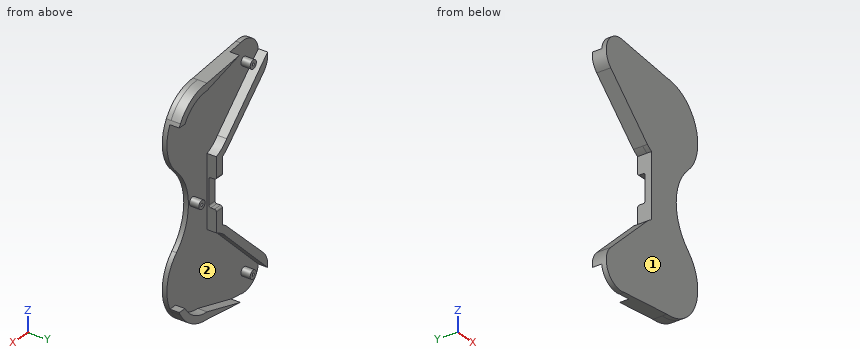
Autodesk Inventor part; units mm, degrees
ref_plane "YZ Plane" through (0, 0, 0) normal (1, 0, 0) x (0, 1, 0)
ref_plane "XZ Plane" through (0, 0, 0) normal (0, 1, 0) x (-1, 0, 0)
ref_plane "XY Plane" through (0, 0, 0) normal (0, 0, 1) x (1, 0, 0)
sketch "Boceto1" plane through (0, 0, 0) normal (0, 1, 0) x (-1, 0, 0)
  line L0 (16, -33) -> (103.2837, -54.9444)
  line L1 (38.5, 50.9711) -> (38.5, 119.0289)
  line L2 (-22.9711, -10.5) -> (-52.9711, -10.5)
  arc A0 (-22.9711, -10.5) -> (16, -33) centre (16, 12) ccw
  arc A1 (-51.515, 38.5517) -> (-6.5, 85) centre (-52.9711, 85) ccw
  arc A2 (-22.9711, -10.5) -> (16, -33) centre (16, 12) ccw
  arc A3 (-51.515, 38.5517) -> (-52.9711, -10.5) centre (16, 12) ccw
  line L3 (38.5, 50.9711) -> (38.5, 85)
  arc A4 (103.2837, -54.9444) -> (115.3375, -21.0974) centre (95.2119, -33) ccw
  line L4 (115.3375, -21.0974) -> (44.6515, 46.7)
  line L5 (16, 203) -> (103.2837, 224.9444)
  arc A5 (16, 203) -> (-22.9711, 180.5) centre (16, 158) ccw
  line L6 (115.3375, 191.0974) -> (44.6515, 123.3)
  arc A6 (115.3375, 191.0974) -> (103.2837, 224.9444) centre (95.2119, 203) ccw
  arc A7 (16, 203) -> (-22.9711, 180.5) centre (16, 158) ccw
  line L7 (38.5, 119.0289) -> (38.5, 50.9711)
  line L8 (-22.9711, 180.5) -> (-52.9711, 180.5)
  line L9 (38.5, 119.0289) -> (38.5, 85)
  arc A8 (-52.9711, 180.5) -> (-51.515, 131.4483) centre (16, 158) ccw
  arc A9 (-6.5, 85) -> (-51.515, 131.4483) centre (-52.9711, 85) ccw
  arc A10 (-22.9711, -10.5) -> (16, -33) centre (16, 12) ccw
  arc A11 (49.4751, 42.0735) -> (38.5, 50.9711) centre (16, 12) ccw
  arc A12 (38.5, 119.0289) -> (49.4751, 127.9265) centre (16, 158) ccw
  arc A13 (16, 203) -> (-22.9711, 180.5) centre (16, 158) ccw
  circle A14 centre (83.6139, -19.9457) radius 1.5
  circle A15 centre (8.5, 85) radius 1.5
  circle A16 centre (83.6139, 189.9457) radius 1.5
  arc A17 (88.6874, -45.3867) -> (105.0119, -23.002) centre (95.2119, -33) ccw
  arc A18 (105.0119, 193.002) -> (91.4604, 216.488) centre (95.2119, 203) ccw
  arc A19 (-48.2434, 32.7133) -> (-48.2434, 137.2867) centre (-52.9711, 85) ccw
  arc A20 (-48.7329, 177.1284) -> (-48.2434, 137.2867) centre (16, 158) ccw
  arc A21 (-48.2434, 32.7133) -> (-48.7329, -7.1284) centre (16, 12) ccw
  line L10 (-48.7329, -7.1284) -> (-16.2545, -7.1284)
  line L11 (-48.7329, 177.1284) -> (-16.2545, 177.1284)
  line L12 (16, 195.5) -> (91.4604, 216.488)
  line L13 (16, -25.5) -> (88.6874, -45.3867)
  line L14 (39.4427, 41.2693) -> (105.0119, -23.002)
  line L15 (105.0119, 193.002) -> (44.7948, 133.9769)
  line L16 (29.5774, 46.9558) -> (29.5774, 123.0442)
  arc A22 (44.7948, 36.0231) -> (29.5774, 46.9558) centre (16, 12) ccw
  arc A23 (-16.2545, -7.1284) -> (16, -25.5) centre (16, 12) ccw
  arc A24 (29.5774, 123.0442) -> (44.7948, 133.9769) centre (16, 158) ccw
  arc A25 (16, 195.5) -> (-16.2545, 177.1284) centre (16, 158) ccw
  circle A26 centre (83.6139, -19.9457) radius 4.5
  circle A27 centre (8.5, 85) radius 4.5
  circle A28 centre (83.6139, 189.9457) radius 4.5
  point P0 (0, 0)
  dimension "d8" = 9
  dimension "d9" = 9
  dimension "d10" = 9
extrude "Extrusión1" add sketch "Boceto1" along normal blind 10 contours A0 L2 A3 A1 A9 A8 L8 A5 L5 A6 L6 A12 L1 A11 L4 A4 L0 | A26 | A27 | A28
sketch "Boceto2" plane through (0, 0, 0) normal (0, -1, 0) x (1, 0, 0)
  line L0 (-16, 203) -> (-103.2837, 224.9444)
  line L1 (22.9711, 180.5) -> (52.9711, 180.5)
  arc A0 (22.9711, 180.5) -> (-16, 203) centre (-16, 158) ccw
  arc A1 (22.9711, 180.5) -> (-16, 203) centre (-16, 158) ccw
  arc A2 (51.515, 131.4483) -> (52.9711, 180.5) centre (-16, 158) ccw
  line L2 (-38.5, 119.0289) -> (-38.5, 85)
  arc A3 (-103.2837, 224.9444) -> (-115.3375, 191.0974) centre (-95.2119, 203) ccw
  line L3 (-115.3375, 191.0974) -> (-44.6515, 123.3)
  line L4 (-16, -33) -> (-103.2837, -54.9444)
  arc A4 (-16, -33) -> (22.9711, -10.5) centre (-16, 12) ccw
  line L5 (-115.3375, -21.0974) -> (-44.6515, 46.7)
  arc A5 (-115.3375, -21.0974) -> (-103.2837, -54.9444) centre (-95.2119, -33) ccw
  arc A6 (-16, -33) -> (22.9711, -10.5) centre (-16, 12) ccw
  line L6 (22.9711, -10.5) -> (52.9711, -10.5)
  line L7 (-38.5, 50.9711) -> (-38.5, 85)
  arc A7 (52.9711, -10.5) -> (51.515, 38.5517) centre (-16, 12) ccw
  arc A8 (51.515, 131.4483) -> (52.9711, 180.5) centre (-16, 158) ccw
  arc A9 (-38.5, 50.9711) -> (-49.4751, 42.0735) centre (-16, 12) ccw
  arc A10 (-16, -33) -> (22.9711, -10.5) centre (-16, 12) ccw
  arc A11 (22.9711, 180.5) -> (-16, 203) centre (-16, 158) ccw
  arc A12 (-49.4751, 127.9265) -> (-38.5, 119.0289) centre (-16, 158) ccw
  arc A13 (51.515, 131.4483) -> (51.515, 38.5517) centre (52.9711, 85) ccw
  arc A14 (51.515, 131.4483) -> (51.515, 38.5517) centre (52.9711, 85) ccw
  point P0 (0, 170)
extrude "Extrusión2" add sketch "Boceto2" along normal blind 5 contours A0 L1 A2 A13 A7 L6 A4 L4 A5 L5 A9 L7 L2 A12 L3 A3 L0
sketch "Boceto3" plane through (-29.5774, 10, 123.0442) normal (1, 0, 0) x (0, 0, -1)
  line L0 (0, 0) -> (76.0885, 0)
  line L1 (38.0442, 0) -> (53.0442, 0)
  line L2 (72.0731, 0) -> (4.0154, 0)
  line L3 (38.0442, 0) -> (23.0442, 0)
  line L4 (23.0442, 0) -> (23.0442, -8)
  line L5 (23.0442, -8) -> (53.0442, -8)
  line L6 (53.0442, -8) -> (53.0442, 0)
  point P0 (123.0442, -10)
  point P1 (53.0442, 0)
  point P2 (23.0442, 0)
  dimension "d15" = 15
  dimension "d16" = 15
  dimension "d17" = 8
extrude "Extrusión3" cut sketch "Boceto3" against normal blind 15
fillet "Empalme1" radius 2 4 edges at (-34.0387, 2, 100) (-34.0387, 2, 70) (-34.0387, 10, 70) (-34.0387, 10, 100)
sketch "Boceto4" plane through (0, 10, 0) normal (0, 1, 0) x (1, 0, 0)
  line L0 (59.5944, 0) -> (46.2124, 0)
  line L1 (46.2124, 0) -> (46.2124, -23.3919)
  line L2 (46.2124, -23.3919) -> (63.6147, -23.3919)
  line L3 (63.6147, -23.3919) -> (63.6147, 0)
  circle A0 centre (-8.5, -85) radius 1.5
  line L4 (-8.5, -85) -> (35.636, -85)
  line L5 (59.5944, -170) -> (46.2124, -170)
  line L6 (46.2124, -170) -> (46.2124, -146.6081)
  line L7 (46.2124, -146.6081) -> (63.6147, -146.6081)
  line L8 (63.6147, -146.6081) -> (63.6147, -170)
  line L9 (59.5944, -170) -> (63.6147, -170)
  line L10 (63.6147, 0) -> (58.9449, 0)
  point P0 (0, 0)
extrude "Extrusión4" cut sketch "Boceto4" against normal blind 8 contours L10 L3 L2 L1 L0 | L5 L6 L7 L8 L9
fillet "Empalme2" radius 2 8 edges at (53.0901, 2, 146.6081) (52.9869, 2, 170) (52.9869, 10, 170) (53.0901, 10, 146.6081) (53.0901, 2, 23.3919) (52.9869, 2, 0) (52.9869, 10, 0) (53.0901, 10, 23.3919)
sketch "Boceto5" plane through (0, 0, 0) normal (0, 1, 0) x (1, 0, 0)
  arc A0 (22.9711, 10.5) -> (-16, 33) centre (-16, -12) ccw
  arc A1 (14.9044, -44.7096) -> (-16, 33) centre (-16, -12) ccw
  arc A2 (6.5, -158) -> (-33.6139, -144) centre (-16, -158) ccw
  arc A3 (14.9044, -44.7096) -> (14.9044, -125.2904) centre (52.9711, -85) ccw
  arc A4 (-78.639, 40.4798) -> (-98.2389, 4.6975) centre (-83.6139, 19.9457) ccw
  arc A5 (-98.2389, -174.6975) -> (-78.639, -210.4798) centre (-83.6139, -189.9457) ccw
  arc A6 (-16, -203) -> (22.9711, -180.5) centre (-16, -158) ccw
  line L0 (-16, -203) -> (-83.6139, -211.0738)
  line L1 (-16, 33) -> (-83.6139, 41.0738)
  arc A7 (-16, -203) -> (14.9044, -125.2904) centre (-16, -158) ccw
  line L2 (-98.2389, 4.6975) -> (-38.5, -52.6001)
  line L3 (-38.5, -119.0289) -> (-38.5, -50.9711)
  line L4 (-98.2389, -174.6975) -> (-38.5, -117.3999)
  line L5 (-38.5, -117.3999) -> (-38.5, -52.6001)
  circle A8 centre (-16, -85) radius 202.8163
  point P0 (0, 0)
  point P1 (-44.6515, -46.7)
  point P2 (-44.6515, -123.3)
extrude "Extrusión5" cut sketch "Boceto5" against normal mid plane 30
properties part number "mando_inf"
Verification items for the finished model (mm, model axes). Face numbers are marked on the shaded views. Coordinates: 2 decimals unless noted, no trailing zeros. Order: outer loops, then holes, each group sorted by start corner. A loop starts at its lowest first (then second) coordinate and runs counter-clockwise, first axis right, second up. Notation, with made-up numbers: (40, -36.5) -> (63, -36.5) arc R11 cw to (63, -31.5) -> close; hole circle Ø10 at (-6.5, -17.5). An arc over 180 degrees is marked (long way). Put each result on its own line as item: value. Start each with the question number.
1. Mould release check, pull along Z, two halves, no side actions. Record for the marked faces 1 and 2: released by +Z, released by -Z, zero draft, split by the parting line, or undercut.
2. Cross-section at A-A, the plane x = -67.5. Record the boundary of the cut face in (y, z), then the cut area to 3 significant figures.
3. Cross-section at C-C, the plane x = 0. Record the boundary of the cut face in (y, z).
4. Go/stop test with flat-tipped pins: pin 1 Ø2.5 at (x, y) = (20.5, 6) entering from -Z; pin 2 Ø5 at (x, y) = (-79.5, 5) entering from +Z; pin 3 Ø4.5 at (x, y) = (-33.5, 6) entering from +Z. Record where each tip stops, or that it passes through.
5. Cross-section at D-D, the plane z = 108.5. Record the boundary of the cut face in (x, y), then the cut area to 3 significant figures.
6. Material ranges on L1, parallel to Z at x = -84, y = 8.5; L2, parallel to X at y = 5, z = 187; L3, parallel to Z at x = -6, y = 0.25, recorded low to high. Write a range as [from, to].
7. Cross-section at B-B, the plane x = -26.5. Record the boundary of the cut face in (y, z), then the cut area to 3 significant figures.
Computed:
1. face 1: zero draft
1. face 2: undercut
2. outline: (-5, -39.15) -> (0, -39.15) -> (0, 13.77) -> (10, 13.77) -> (10, 24.79) -> (-5, 24.79) -> close; (-5, 145.21) -> (10, 145.21) -> (10, 156.23) -> (0, 156.23) -> (0, 209.15) -> (-5, 209.15) -> close
2. area: 860 mm2
3. outline: (-5, -30.06) -> (10, -30.06) -> (10, -21.92) -> (0, -21.92) -> (0, 68.68) -> (-5, 68.68) -> close; (-5, 101.32) -> (0, 101.32) -> (0, 191.92) -> (10, 191.92) -> (10, 200.06) -> (-5, 200.06) -> close
4. pin 1: z = -15.97
4. pin 2: z = 194.15
4. pin 3: z = 205.36
5. outline: (-38.5, -5) -> (2.77, -5) -> (2.77, 0) -> (-29.58, 0) -> (-29.58, 10) -> (-38.5, 10) -> close
5. area: 296 mm2
6. L1: [-24.43, -21.4], [-18.5, -15.46], [-2.41, 8.96], [161.04, 172.41], [185.46, 188.5], [191.4, 194.43]
6. L2: [-104.54, -98.89], [-87.02, -80.21], [7.77, 18.41]
6. L3: [-31.87, -24.14], [81.26, 88.74], [194.14, 201.87]
7. outline: (-5, -34.25) -> (10, -34.25) -> (10, -28.37) -> (0, -28.37) -> (0, 198.42) -> (10, 198.42) -> (10, 204.25) -> (-5, 204.25) -> close
7. area: 1,310 mm2
